```python
from build123d import *

# Parameters (mm, degrees)
SKETCH1_W           = 20
SKETCH1_H           = 200
SKETCH1_R           = 2.5
BOSS_EXTRUDE1_DEPTH = 20
CHAMFER1_SIZE       = 10
SCALE1_SCALE        = 7.5


with BuildPart() as part:
    # Sketch1 → Boss-Extrude1 (new body)
    with BuildSketch(Plane(origin=(0, 0, 0), x_dir=(1, 0, 0), z_dir=(0, 1, 0))):
        with Locations((10, -100)):
            Rectangle(SKETCH1_W, SKETCH1_H)
        with Locations(Location((10, -10, 0), (0, 0, 270))):
            Circle(SKETCH1_R, mode=Mode.SUBTRACT)
        with Locations(Location((10, -70, 0), (0, 0, 270))):
            Circle(SKETCH1_R, mode=Mode.SUBTRACT)
    extrude(amount=BOSS_EXTRUDE1_DEPTH)

    # Chamfer1
    chamfer1_edges = [part.edges().sort_by_distance(p)[0] for p in [
        (10, 0, 200),
        (10, 20, 200),
        (20, 10, 200),
        (0, 10, 200),
    ]]
    chamfer(chamfer1_edges, length=CHAMFER1_SIZE - 0.0001)  # a hair under: the kernel refuses the full size


with BuildPart() as part_1:
    # Scale1: scaled about (10, 10, 97.262644204)
    add(part.part.scale(SCALE1_SCALE).moved(Location((-65, -65, -632.207187326))))


solid = part_1.part
```
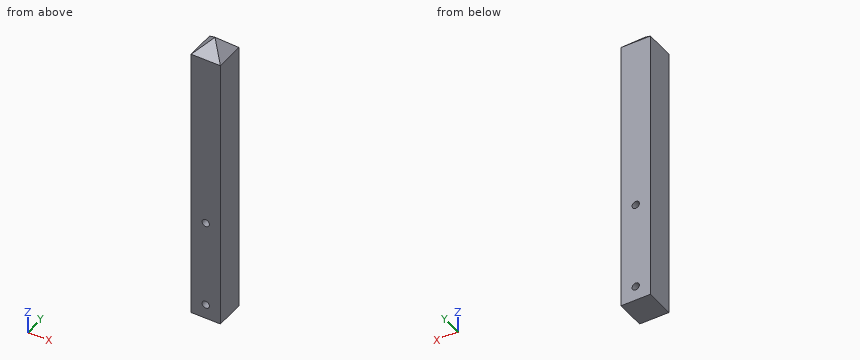
Here's how the part is built. I have some questions about the finished solid (model axes, mm). Coordinates: 2 decimals unless noted, no trailing zeros. Loops run counter-clockwise (first coordinate to the right, second up) from the corner with the lowest first, then second, coordinate; pieces in that order, holes last. Notation, with made-up numbers: (83.5, 6) - (91.5, 6) arc R14 ccw to (91.5, 10) - close; hole circle Ø1 at (34, -12.75). An arc over 180 degrees is marked (long way). Return JSON: item names as keys, results as strings. Group by question number.
Item 1: I need wall thicknesses on line 1 (Z direction, x = 24, y = 38); line 2 (X direction, y = 16.5, z = -558.5); line 3 (Z direction, x = -25.5, y = -46). Which ranges of each line are inside material? Lowest first, please. Write a range as from..to.
Item 2: If we section it at C-C on x = -40: Write out the boundary of the cut face in (y, z).
Item 3: If we section it at B-B on y = -43: Write out the boundary of the cut face in (x, z).
Item 4: If we section it at A-A on y = 23: Write out the boundary of the cut face in (x, z), and give its area (3 significant figures).
Calculated:
{
 "1": {"line 1": "z = -632.21..-569.68, -544.73..-119.68, -94.73..839.79", "line 2": "x = -65..-8.71, 28.71..85", "line 3": "z = -632.21..811.79"},
 "2": {"outline": "(-65, -632.21) - (85, -632.21) - (85, 792.79) - (60, 817.79) - (-40, 817.79) - (-65, 792.79) - close"},
 "3": {"outline": "(-65, -632.21) - (85, -632.21) - (85, 792.79) - (63, 814.79) - (-43, 814.79) - (-65, 792.79) - close; hole circle Ø37.5 at (10, -557.21); hole circle Ø37.5 at (10, -107.21)"},
 "4": {"outline": "(-65, -632.21) - (85, -632.21) - (85, 792.79) - (23, 854.79) - (-3, 854.79) - (-65, 792.79) - close; hole circle Ø37.5 at (10, -557.21); hole circle Ø37.5 at (10, -107.21)", "area": "217,000 mm^2"}
}
